Answer from the drawing. Dimensions are ordinates in mm from the lowest x, y and z of the part. A direction names the side the tool comes from. Round coordinates to 2 decimals unless told otherwise and drop trailing zeros. Write each loop counter-clockwise with the first axis right and the second up, starting at its lowest first coordinate (ties: lowest second). Pieces come first, ordered by that corner, then holes. Notation, with made-up numbers: (15, -34.5) -> (73, -34.5) arc R23 cw to (73, -6.5) -> close; hole circle Ø9 at (-4, -30). An arc over 180 degrees is marked (long way). Answer as a JSON object with one key per item and string values. Group by question number.
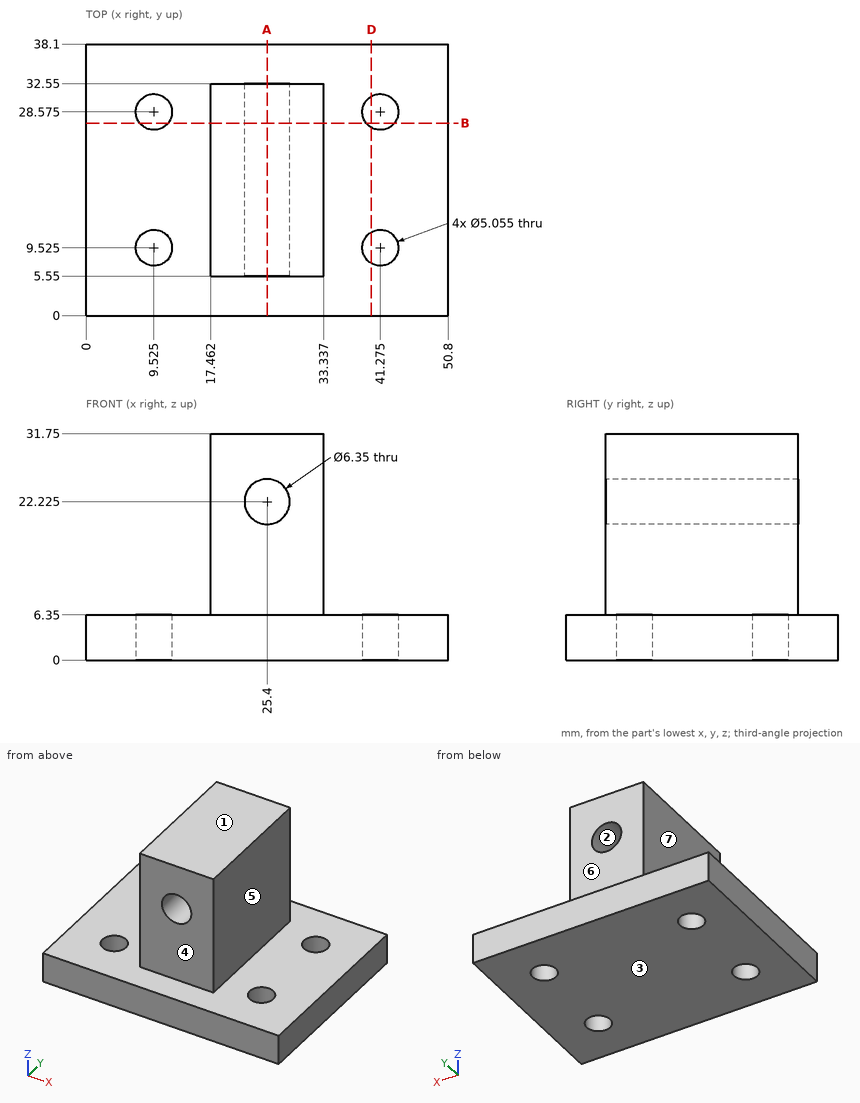
1) Straight lines are drawn through the part: L1, parallel to Y at x = 43, z = 4.5; L2, parallel to Z at x = 25.4, y = 19; L3, parallel to Z at x = 40, y = 20. For each, find the intervals that lie inside material, in ascending order.
2) For a pull along Z with two mould halves and no side action, classify the marked faces 1, 2, 3 and 4 as released by +Z, released by -Z, zero draft, split by the parting line, or undercut.
3) A cutting plane is placed at D-D on x = 40. Determine the outline of the cut face in (y, z).
4) Each of these flat-tipped pins is pushed along its axis until it touches: P1, Ø4, axis at x = 9.525, y = 9.525, coming from the -Z side; P2, Ø12, axis at y = 14, z = 12, coming from the -X side; P3, Ø8, axis at x = 41.275, y = 28.575, coming from the +Z side; P4, Ø8, axis at x = 27.5, z = 17, coming from the +Y side. Where does it stop, or does it pass through?
5) A tool of negligible diameter and unlimited length cuts with its end or side. For the marked faces 5, 6 and 7, from which of +Z, -Z, +X, -X, +Y, -Y can it reach the whole face along a straight path? Write none if from no direction.
6) A cutting plane is placed at B-B on y = 27. State how many separate pieces and enclosed holes the cut face has, plus the area to 3 significant figures.
7) A cutting plane is placed at A-A on x = 25.4. Determine the outline of the cut face in (y, z).
Established:
{
 "1": {"L1": "y = 0 to 7.68, 11.37 to 26.73, 30.42 to 38.1", "L2": "z = 0 to 19.05, 25.4 to 31.75", "L3": "z = 0 to 6.35"},
 "2": {"face 1": "released by +Z", "face 2": "undercut", "face 3": "released by -Z", "face 4": "zero draft"},
 "3": {"outline": "(0, 0) -> (7.34, 0) -> (7.34, 6.35) -> (0, 6.35) -> close; (11.71, 0) -> (26.39, 0) -> (26.39, 6.35) -> (11.71, 6.35) -> close; (30.76, 0) -> (38.1, 0) -> (38.1, 6.35) -> (30.76, 6.35) -> close"},
 "4": {"P1": "passes through", "P2": "stops at x = 0", "P3": "stops at z = 6.35", "P4": "stops at y = 32.55"},
 "5": {"face 5": "+Z, +X, +Y, -Y", "face 6": "+Z, +X, -X, +Y", "face 7": "+Z, -X, +Y, -Y"},
 "6": {"separate pieces": "3", "enclosed holes": "1", "area": "644 mm²"},
 "7": {"outline": "(0, 0) -> (38.1, 0) -> (38.1, 6.35) -> (32.55, 6.35) -> (32.55, 19.05) -> (5.55, 19.05) -> (5.55, 6.35) -> (0, 6.35) -> close; (5.55, 25.4) -> (32.55, 25.4) -> (32.55, 31.75) -> (5.55, 31.75) -> close"}
}
